Check sheet for the modelled part. Datum: model origin and axes. Units: mm. Coordinates: 2 decimals unless noted, no trailing zeros. Loops run counter-clockwise (first coordinate to the right, second up) from the corner with the lowest first, then second, coordinate; pieces in that order, holes last. Notation, with made-up numbers: M 72.25,12.5 L 102.25,12.5 A24 ccw 102.25,36.5 Z; hole C 39,21.5 d8. An arc over 180 degrees is marked long. Use CSV: the item, a comma, the result in double quotes. Start each with the question number.
(1) Section check B-B on y = 0.65. Give the number of separate pieces and of enclosed holes in the cut face, and give its area (3 significant figures).
(2) Section check A-A on x = 10. Record the cut outline in (y, z) (3 decimals), and give its area (3 significant figures).
(3) Scan lines: line 1 (Z direction, x = 74.5, y = 1.2); line 2 (Z direction, x = 80, y = 1.6); line 3 (Z direction, x = -12.5, y = 1.4). Record each from-to range of solid material in increasing order.
from build123d import *

# Parameters (mm, degrees)
SKETCH1_W           = 215
SKETCH1_H           = 110
BOSS_EXTRUDE1_DEPTH = 3.175
SKETCH2_W           = 147
SKETCH2_H           = 37
CUT_EXTRUDE1_DEPTH  = 121.79458028
SKETCH3_W           = 7.9
SKETCH3_H           = 40
CUT_EXTRUDE2_DEPTH  = 121.79458028
SKETCH5_R           = 1.6
CUT_EXTRUDE4_DEPTH  = 121.79458028
SKETCH6_R           = 1.6
CUT_EXTRUDE5_DEPTH  = 121.79458028
CUT_EXTRUDE6_DEPTH  = 121.79458028
FILLET1_R           = 3


with BuildPart() as part:
    # Sketch1 → Boss-Extrude1 (new body)
    with BuildSketch(Plane(origin=(0, 0, 0), x_dir=(1, 0, 0), z_dir=(0, 1, 0))):
        Rectangle(SKETCH1_W, SKETCH1_H)
    extrude(amount=BOSS_EXTRUDE1_DEPTH)

    # Sketch2 → Cut-Extrude1 (cut, through all)
    with BuildSketch(Plane.XZ):
        Rectangle(SKETCH2_W, SKETCH2_H)
    extrude(amount=-CUT_EXTRUDE1_DEPTH, mode=Mode.SUBTRACT)

    # Sketch3 → Cut-Extrude2 (cut, through all)
    with BuildSketch(Plane(origin=(0, 3.175, 0), x_dir=(1, 0, 0), z_dir=(0, 1, 0))):
        with Locations((-103.55, 0)):
            Rectangle(SKETCH3_W, SKETCH3_H)
    extrude(amount=-CUT_EXTRUDE2_DEPTH, mode=Mode.SUBTRACT)

    # Sketch5 → Cut-Extrude4 (cut, through all)
    with BuildSketch(Plane(origin=(0, 3.175, 0), x_dir=(1, 0, 0), z_dir=(0, 1, 0))):
        with Locations(Location((80, 25, 0), (0, 0, 270))):
            Circle(SKETCH5_R)
        with Locations(Location((80, -25, 0), (0, 0, 270))):
            Circle(SKETCH5_R)
        with Locations(Location((0, 25, 0), (0, 0, 270))):
            Circle(SKETCH5_R)
        with Locations(Location((0, -25, 0), (0, 0, 270))):
            Circle(SKETCH5_R)
        with Locations(Location((-80, 25, 0), (0, 0, 270))):
            Circle(SKETCH5_R)
        with Locations(Location((-80, -25, 0), (0, 0, 270))):
            Circle(SKETCH5_R)
    extrude(amount=-CUT_EXTRUDE4_DEPTH, mode=Mode.SUBTRACT)

    # Sketch6 → Cut-Extrude5 (cut, through all)
    with BuildSketch(Plane(origin=(0, 3.175, 0), x_dir=(1, 0, 0), z_dir=(0, 1, 0))):
        with Locations(Location((-74.528255169, -42.068885296, 0), (0, 0, 270))):
            Circle(SKETCH6_R)
        with Locations(Location((-37.528255169, -42.068885296, 0), (0, 0, 270))):
            Circle(SKETCH6_R)
        with Locations(Location((0, -42.068885296, 0), (0, 0, 270))):
            Circle(SKETCH6_R)
        with Locations(Location((37.528255169, -42.068885296, 0), (0, 0, 90))):
            Circle(SKETCH6_R)
        with Locations(Location((74.528255169, -42.068885296, 0), (0, 0, 90))):
            Circle(SKETCH6_R)
        with Locations(Location((74.528255169, 42.068885296, 0), (0, 0, 270))):
            Circle(SKETCH6_R)
        with Locations(Location((37.528255169, 42.068885296, 0), (0, 0, 270))):
            Circle(SKETCH6_R)
        with Locations(Location((0, 42.068885296, 0), (0, 0, 90))):
            Circle(SKETCH6_R)
        with Locations(Location((-37.528255169, 42.068885296, 0), (0, 0, 90))):
            Circle(SKETCH6_R)
        with Locations(Location((-74.528255169, 42.068885296, 0), (0, 0, 90))):
            Circle(SKETCH6_R)
    extrude(amount=-CUT_EXTRUDE5_DEPTH, mode=Mode.SUBTRACT)

    # Sketch7 → Cut-Extrude6 (cut, through all)
    with BuildSketch(Plane(origin=(0, 3.175, 0), x_dir=(1, 0, 0), z_dir=(0, 1, 0))):
        Polygon((-88.5, 46.725), (-87.4, 46.725), (-87.4, 50.1), (-88.5, 50.1), (-101.5, 50.1), (-102.6, 50.1), (-102.6, 46.725), (-101.5, 46.725), align=None)
        Polygon((-102.6, 33.55), (-101.5, 33.55), (-88.5, 33.55), (-87.4, 33.55), (-87.4, 36.925), (-88.5, 36.925), (-101.5, 36.925), (-102.6, 36.925), align=None)
        Polygon((-88.5, -36.925), (-87.4, -36.925), (-87.4, -33.55), (-88.5, -33.55), (-101.5, -33.55), (-102.6, -33.55), (-102.6, -36.925), (-101.5, -36.925), align=None)
        Polygon((-102.6, -50.1), (-101.5, -50.1), (-88.5, -50.1), (-87.4, -50.1), (-87.4, -46.725), (-88.5, -46.725), (-101.5, -46.725), (-102.6, -46.725), align=None)
    extrude(amount=-CUT_EXTRUDE6_DEPTH, mode=Mode.SUBTRACT)

    # Fillet1
    fillet1_edges = [part.edges().sort_by_distance(p)[0] for p in [
        (-73.5, 1.5875, -18.5),
        (-73.5, 1.5875, 18.5),
        (73.5, 1.5875, 18.5),
        (73.5, 1.5875, -18.5),
        (-99.6, 1.5875, -20),
        (-99.6, 1.5875, 20),
        (-107.5, 1.5875, 20),
        (-107.5, 1.5875, -20),
        (-107.5, 1.5875, -55),
        (107.5, 1.5875, -55),
        (107.5, 1.5875, 55),
        (-107.5, 1.5875, 55),
    ]]
    fillet(fillet1_edges, radius=FILLET1_R)


solid = part.part
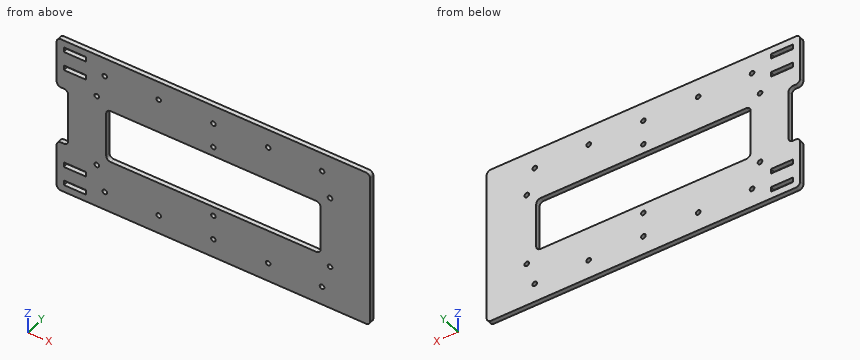
Outcome:
1,separate pieces,"1"
1,enclosed holes,"21"
1,area,"17,600 mm²"
2,outline,"M 0,-55 L 3.175,-55 L 3.175,-18.5 L 0,-18.5 Z; M 0,18.5 L 3.175,18.5 L 3.175,55 L 0,55 Z"
2,area,"232 mm²"
3,line 1,"z = -55 to -43.67, -40.47 to 40.47, 43.67 to 55"
3,line 2,"z = -55 to -26.6, -23.4 to 23.4, 26.6 to 55"
3,line 3,"z = -55 to -18.5, 18.5 to 55"
